from build123d import *

# Parameters (mm, degrees)
SKETCH1_W                         = 50.8
SKETCH1_H                         = 44.45
EXTRUDE1_DEPTH                    = 6.35
F_1_4_20_TAPPED_HOLE1_D           = 5.1054
F_1_4_20_TAPPED_HOLE1_DEPTH       = 14.9098
F_1_4_20_TAPPED_HOLE1_CSINK_D     = 8.3312
F_1_4_20_TAPPED_HOLE1_CSINK_ANGLE = 82
F_1_4_20_TAPPED_HOLE1_TIP         = 1.533816902
F_1_4_20_TAPPED_HOLE2_D           = 5.1054
F_1_4_20_TAPPED_HOLE2_DEPTH       = 16.51
F_1_4_20_TAPPED_HOLE2_TIP         = 1.533816902


with BuildPart() as part:
    # Sketch1 → Extrude1 (new, symmetric)
    with BuildSketch(Plane(origin=(0, 0, 0), x_dir=(0, 0, -1), z_dir=(1, 0, 0))):
        with Locations((-9.525, 3.175)):
            Rectangle(SKETCH1_W, SKETCH1_H)
    extrude(amount=EXTRUDE1_DEPTH, both=True)

    # 1/4-20 Tapped Hole1
    with Locations(Plane.XZ.offset(19.05)):
        with Locations((0, 26.035), (0, -5.715)):
            CounterSinkHole(F_1_4_20_TAPPED_HOLE1_D / 2, F_1_4_20_TAPPED_HOLE1_CSINK_D / 2, depth=F_1_4_20_TAPPED_HOLE1_DEPTH, counter_sink_angle=F_1_4_20_TAPPED_HOLE1_CSINK_ANGLE)
            with Locations((0, 0, -(F_1_4_20_TAPPED_HOLE1_DEPTH + F_1_4_20_TAPPED_HOLE1_TIP / 2))):  # 118° drill point
                Cone(0, F_1_4_20_TAPPED_HOLE1_D / 2, F_1_4_20_TAPPED_HOLE1_TIP, mode=Mode.SUBTRACT)

    # 1/4-20 Tapped Hole2
    with Locations(Plane(origin=(0, 25.4, 0), x_dir=(-1, 0, 0), z_dir=(0, 1, 0))):
        with Locations((0, 9.525)):
            Hole(F_1_4_20_TAPPED_HOLE2_D / 2, depth=F_1_4_20_TAPPED_HOLE2_DEPTH)
            with Locations((0, 0, -(F_1_4_20_TAPPED_HOLE2_DEPTH + F_1_4_20_TAPPED_HOLE2_TIP / 2))):  # 118° drill point
                Cone(0, F_1_4_20_TAPPED_HOLE2_D / 2, F_1_4_20_TAPPED_HOLE2_TIP, mode=Mode.SUBTRACT)


solid = part.part
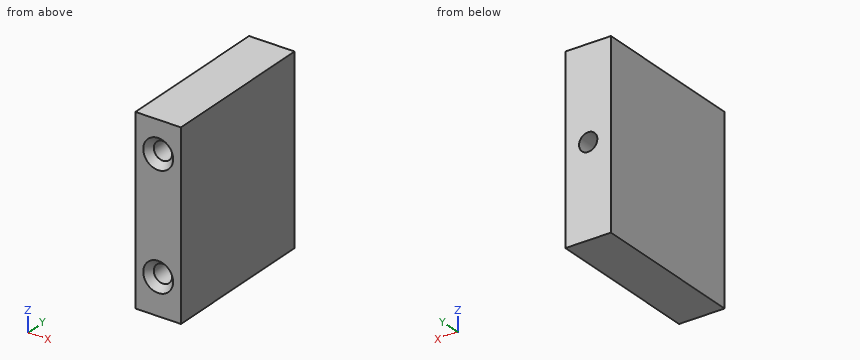
CAD build for the part. Positions are in the model's coordinates, mm. Round coordinates to 2 decimals unless told otherwise and drop trailing zeros. Loops run counter-clockwise (first coordinate to the right, second up) from the corner with the lowest first, then second, coordinate; pieces in that order, holes last. Notation, with made-up numbers: (2, -3) - (57, -3) arc R19 ccw to (57, 18) - close; hole circle Ø7 at (72.5, 14.25). An arc over 180 degrees is marked (long way). Put each result on its own line as item: value.
1. Slice it at B-B on y = -11.5. List the corners of the cut face in (x, z) (3 decimals), and give its area (3 significant figures).
Geometry check:
outline: (-6.35, -15.875) - (6.35, -15.875) - (6.35, 34.925) - (-6.35, 34.925) - close; hole circle Ø5.105 at (0, -5.715); hole circle Ø5.105 at (0, 26.035)
area: 604 mm²
2. Wall check: line 1 (Z direction, x = 0, y = -12) (3 decimals); line 2 (Z direction, x = 0, y = 22.25) (3 decimals); line 3 (X direction, y = 16, z = 9.5). Give the ranges that are in metal, low to high.
Geometry check:
line 1: -15.875 to -8.268, -3.162 to 23.482, 28.588 to 34.925
line 2: -15.875 to 6.972, 12.078 to 34.925
line 3: -6.35 to -2.55, 2.55 to 6.35
3. Slice it at A-A on y = 20. List the corners of the cut face in (x, z) (3 decimals).
Geometry check:
outline: (-6.35, -15.875) - (6.35, -15.875) - (6.35, 34.925) - (-6.35, 34.925) - close; hole circle Ø5.105 at (0, 9.525)
4. Pin check, flat tips, straight feed: P1, Ø1, axis at x = -2.5, z = -6.5, coming from the -Y side; P2, Ø3, axis at x = 0, z = 26.035, coming from the -Y side; P3, Ø4.5, axis at x = 0, z = 9.525, coming from the +Y side. Stop position of each tip, or through.
Geometry check:
P1: y = -17.85
P2: y = -3.51
P3: y = 8.71
